Design review of the part built by this model. Coordinates are the model's own, in mm. A direction names the side the tool comes from. Round coordinates to 2 decimals unless told otherwise and drop trailing zeros. Loops run counter-clockwise (first coordinate to the right, second up) from the corner with the lowest first, then second, coordinate; pieces in that order, holes last. Notation, with made-up numbers: (36, 89) - (56, 89) arc R24 ccw to (56, 110) - close; hole circle Ø3 at (75, 78.5). An arc over 180 degrees is marked (long way). Answer as CSV lines item,"result". Start each with the question number.
(1) Consider section A-A (x = 23.75). Give the boundary of the cut face in (y, z), and give its area (3 significant figures).
(2) Consider section B-B (z = -1.75). Give the boundary of the cut face in (x, y), and give its area (3 significant figures).
(3) Consider section C-C (y = -14.25). Give the boundary of the cut face in (x, z).
(4) Mouldability with a two-part tool opening along X and no side actions: class faces 5 (the cylindrical face through (-21.461, -3.074, -0.14)), 6 (the flat face through (26, -3, 0)), 7 (the flat face through (11, -5, -7)) as released by +X, released by -X, zero draft, split by the parting line, or undercut.
(5) For P1, Ø3, axis at x = -9.5, z = -5.5, coming from the +Y side; P2, Ø2, axis at y = -22, z = 0.5, coming from the -X side; P3, Ø1, axis at x = 15.5, z = -3, coming from the +Y side; P4, Ø1.5, axis at x = -13, z = -8, coming from the -Y side, all flat-tipped, find the tip position at first contact; note any pin that passes through.
(6) For faces 1 (the flat face through (0, -25, 0)), 2 (the flat face through (-14, -8, 8)), 3 (the cylindrical face through (-5.85, -5.57, -7.46)), 4 (the flat face through (-7, -12, 0)), list the 3-axis set-ups (+Z, -Z, +X, -X, +Y, -Y) from which the entire face can be reached by the end or side of a thin tool; tool diameter is ignored.
(7) Consider section D-D (x = -23). Give the boundary of the cut face in (y, z).
(8) Wall thickness on L1, parallel to Z at x = -23.75, y = -1.7; L2, parallel to X at y = -1.15, z = -4.75; L3, parallel to X at y = -15.5, z = 4: over which ranges is each line inside the solid? List them lowest first.
from build123d import *

# Parameters (mm, degrees)
BOSS_EXTRUDE1_DEPTH = 10
SKETCH2_R           = 2
CUT_EXTRUDE1_DEPTH  = 6
SKETCH3_W           = 10
SKETCH3_H           = 12
CUT_EXTRUDE2_DEPTH  = 21
FILLET1_R           = 2


with BuildPart() as part:
    # Sketch1 → Boss-Extrude1 (new, symmetric)
    with BuildSketch(Plane.XY):
        Polygon((-30, 0), (-17, 0), (-17, -5), (-5.25, -5), (-5.25, -22), (5.25, -22), (5.25, -5), (17, -5), (17, 0), (30, 0), (30, -3), (20, -3), (20, -8), (8.25, -8), (8.25, -25), (-8.25, -25), (-8.25, -8), (-20, -8), (-20, -3), (-30, -3), align=None)
    extrude(amount=BOSS_EXTRUDE1_DEPTH, both=True)

    # Sketch2 → Cut-Extrude1 (cut)
    with BuildSketch(Plane(origin=(0, 0, 0), x_dir=(1, 0, 0), z_dir=(0, 1, 0))):
        with Locations(Location((-23.75, 4.75, 0), (0, 0, 270))):
            Circle(SKETCH2_R)
        with Locations(Location((-23.75, -4.75, 0), (0, 0, 270))):
            Circle(SKETCH2_R)
        with Locations(Location((23.75, 4.75, 0), (0, 0, 270))):
            Circle(SKETCH2_R)
        with Locations(Location((23.75, -4.75, 0), (0, 0, 270))):
            Circle(SKETCH2_R)
    extrude(amount=-CUT_EXTRUDE1_DEPTH, mode=Mode.SUBTRACT)

    # Sketch3 → Cut-Extrude2 (cut, symmetric)
    with BuildSketch(Plane(origin=(0, 0, 0), x_dir=(0, 0, -1), z_dir=(1, 0, 0))):
        with Locations((0, -6)):
            Rectangle(SKETCH3_W, SKETCH3_H)
    extrude(amount=CUT_EXTRUDE2_DEPTH, both=True, mode=Mode.SUBTRACT)

    # Fillet1
    # the kernel refuses this fillet: 2 mm, written as the material it adds along each edge
    with BuildSketch(Plane(origin=(-17, -5, 10), x_dir=(0, 1, 0), z_dir=(0, 0, -1)), Plane(origin=(17, -5, 10), x_dir=(-1, 0, 0), z_dir=(0, 0, -1)), Plane(origin=(8.25, -8, 10), x_dir=(1, 0, 0), z_dir=(0, 0, -1)), Plane(origin=(-8.25, -8, 10), x_dir=(0, -1, 0), z_dir=(0, 0, -1)), Plane(origin=(-17, -5, -5), x_dir=(0, 1, 0), z_dir=(0, 0, -1)), Plane(origin=(17, -5, -5), x_dir=(-1, 0, 0), z_dir=(0, 0, -1)), Plane(origin=(-8.25, -8, -5), x_dir=(0, -1, 0), z_dir=(0, 0, -1))) as fillet1_piece_1:
        with BuildLine():
            CenterArc((FILLET1_R, FILLET1_R), FILLET1_R, 180, 90)
            Line((0, FILLET1_R), (0, 0))
            Line((0, 0), (FILLET1_R, 0))
        make_face()
    extrude(amount=5)
    with BuildSketch(Plane(origin=(-5.25, -22, 10), x_dir=(0, 1, 0), z_dir=(0, 0, -1)), Plane(origin=(5.25, -22, 10), x_dir=(-1, 0, 0), z_dir=(0, 0, -1))) as fillet1_piece_2:
        with BuildLine():
            CenterArc((FILLET1_R, FILLET1_R), FILLET1_R, 180, 90)
            Line((0, FILLET1_R), (0, 0))
            Line((0, 0), (FILLET1_R, 0))
        make_face()
    extrude(amount=20)
    with BuildSketch(Plane(origin=(20, -3, 10), x_dir=(1, 0, 0), z_dir=(0, 0, -1))) as fillet1_piece_3_section:
        with BuildLine():
            CenterArc((FILLET1_R, FILLET1_R), FILLET1_R, 180, 90)
            Line((0, FILLET1_R), (0, 0))
            Line((0, 0), (FILLET1_R, 0))
        make_face()
    fillet1_piece_3 = extrude(amount=5, mode=Mode.PRIVATE)
    fillet1_piece_3 = split(fillet1_piece_3, bisect_by=Plane(origin=(21, -3.048479196, 7.515597856), z_dir=(1, 0, 0)), keep=Keep.TOP, mode=Mode.PRIVATE)
    fillet1_piece_3 = fillet1_piece_3 - Plane(origin=(23.75, -3.048479196, 4.75), x_dir=(0, 0, 1), z_dir=(0, 1, 0)) * Cylinder(2, 18, mode=Mode.PRIVATE)
    add(fillet1_piece_3)
    with BuildSketch(Plane(origin=(20, -3, 10), x_dir=(1, 0, 0), z_dir=(0, 0, -1))) as fillet1_piece_4_section:
        with BuildLine():
            CenterArc((FILLET1_R, FILLET1_R), FILLET1_R, 180, 90)
            Line((0, FILLET1_R), (0, 0))
            Line((0, 0), (FILLET1_R, 0))
        make_face()
    fillet1_piece_4 = extrude(amount=5, mode=Mode.PRIVATE)
    fillet1_piece_4 = split(fillet1_piece_4, bisect_by=Plane(origin=(21, -3.51024012, 7.5), z_dir=(-1, 0, 0)), keep=Keep.TOP, mode=Mode.PRIVATE)
    add(fillet1_piece_4)
    with BuildSketch(Plane(origin=(20, -3, 10), x_dir=(1, 0, 0), z_dir=(0, 0, -1))) as fillet1_piece_5_section:
        with BuildLine():
            CenterArc((FILLET1_R, FILLET1_R), FILLET1_R, 180, 90)
            Line((0, FILLET1_R), (0, 0))
            Line((0, 0), (FILLET1_R, 0))
        make_face()
    fillet1_piece_5 = extrude(amount=10, mode=Mode.PRIVATE)
    fillet1_piece_5 = split(fillet1_piece_5, bisect_by=Plane(origin=(21.317615257, -3.049059645, 5), z_dir=(0, 0, -1)), keep=Keep.TOP, mode=Mode.PRIVATE)
    fillet1_piece_5 = split(fillet1_piece_5, bisect_by=Plane(origin=(21, -3.049059645, 2.467907611), z_dir=(1, 0, 0)), keep=Keep.TOP, mode=Mode.PRIVATE)
    fillet1_piece_5 = fillet1_piece_5 - Plane(origin=(23.75, -3.049059645, 4.75), x_dir=(0, 0, 1), z_dir=(0, 1, 0)) * Cylinder(2, 28, mode=Mode.PRIVATE)
    add(fillet1_piece_5)
    with BuildSketch(Plane(origin=(-20, -3, 0), x_dir=(-1, 0, 0), z_dir=(0, 0, 1))) as fillet1_piece_6_section:
        with BuildLine():
            CenterArc((FILLET1_R, FILLET1_R), FILLET1_R, 180, 90)
            Line((0, FILLET1_R), (0, 0))
            Line((0, 0), (FILLET1_R, 0))
        make_face()
    fillet1_piece_6 = extrude(amount=10, mode=Mode.PRIVATE)
    fillet1_piece_6 = split(fillet1_piece_6, bisect_by=Plane(origin=(-21.317615257, -3.049059645, 5), z_dir=(0, 0, -1)), keep=Keep.TOP, mode=Mode.PRIVATE)
    fillet1_piece_6 = split(fillet1_piece_6, bisect_by=Plane(origin=(-21, -3.049059645, 2.46790761), z_dir=(-1, 0, 0)), keep=Keep.TOP, mode=Mode.PRIVATE)
    fillet1_piece_6 = fillet1_piece_6 - Plane(origin=(-23.75, -3.049059645, 4.75), x_dir=(0, 0, 1), z_dir=(0, 1, 0)) * Cylinder(2, 28, mode=Mode.PRIVATE)
    add(fillet1_piece_6)
    with BuildSketch(Plane(origin=(-20, -3, 5), x_dir=(-1, 0, 0), z_dir=(0, 0, 1))) as fillet1_piece_7_section:
        with BuildLine():
            CenterArc((FILLET1_R, FILLET1_R), FILLET1_R, 180, 90)
            Line((0, FILLET1_R), (0, 0))
            Line((0, 0), (FILLET1_R, 0))
        make_face()
    fillet1_piece_7 = extrude(amount=5, mode=Mode.PRIVATE)
    fillet1_piece_7 = split(fillet1_piece_7, bisect_by=Plane(origin=(-21, -3.048479196, 7.515597855), z_dir=(-1, 0, 0)), keep=Keep.TOP, mode=Mode.PRIVATE)
    fillet1_piece_7 = fillet1_piece_7 - Plane(origin=(-23.75, -3.048479196, 4.75), x_dir=(0, 0, 1), z_dir=(0, 1, 0)) * Cylinder(2, 18, mode=Mode.PRIVATE)
    add(fillet1_piece_7)
    with BuildSketch(Plane(origin=(-20, -3, 5), x_dir=(-1, 0, 0), z_dir=(0, 0, 1))) as fillet1_piece_8_section:
        with BuildLine():
            CenterArc((FILLET1_R, FILLET1_R), FILLET1_R, 180, 90)
            Line((0, FILLET1_R), (0, 0))
            Line((0, 0), (FILLET1_R, 0))
        make_face()
    fillet1_piece_8 = extrude(amount=5, mode=Mode.PRIVATE)
    fillet1_piece_8 = split(fillet1_piece_8, bisect_by=Plane(origin=(-21, -3.51024012, 7.5), z_dir=(1, 0, 0)), keep=Keep.TOP, mode=Mode.PRIVATE)
    add(fillet1_piece_8)
    with BuildSketch(Plane(origin=(20, -3, 0), x_dir=(1, 0, 0), z_dir=(0, 0, -1))) as fillet1_piece_9_section:
        with BuildLine():
            CenterArc((FILLET1_R, FILLET1_R), FILLET1_R, 180, 90)
            Line((0, FILLET1_R), (0, 0))
            Line((0, 0), (FILLET1_R, 0))
        make_face()
    fillet1_piece_9 = extrude(amount=10, mode=Mode.PRIVATE)
    fillet1_piece_9 = split(fillet1_piece_9, bisect_by=Plane(origin=(21, -3.049059645, -2.46790761), z_dir=(1, 0, 0)), keep=Keep.TOP, mode=Mode.PRIVATE)
    fillet1_piece_9 = split(fillet1_piece_9, bisect_by=Plane(origin=(21.317615257, -3.049059645, -5), z_dir=(0, 0, 1)), keep=Keep.TOP, mode=Mode.PRIVATE)
    fillet1_piece_9 = fillet1_piece_9 - Plane(origin=(23.75, -3.049059645, -4.75), x_dir=(0, 0, 1), z_dir=(0, 1, 0)) * Cylinder(2, 28, mode=Mode.PRIVATE)
    add(fillet1_piece_9)
    with BuildSketch(Plane(origin=(20, -3, -5), x_dir=(1, 0, 0), z_dir=(0, 0, -1))) as fillet1_piece_10_section:
        with BuildLine():
            CenterArc((FILLET1_R, FILLET1_R), FILLET1_R, 180, 90)
            Line((0, FILLET1_R), (0, 0))
            Line((0, 0), (FILLET1_R, 0))
        make_face()
    fillet1_piece_10 = extrude(amount=5, mode=Mode.PRIVATE)
    fillet1_piece_10 = split(fillet1_piece_10, bisect_by=Plane(origin=(21, -3.048479196, -7.515597854), z_dir=(1, 0, 0)), keep=Keep.TOP, mode=Mode.PRIVATE)
    fillet1_piece_10 = fillet1_piece_10 - Plane(origin=(23.75, -3.048479196, -4.75), x_dir=(0, 0, 1), z_dir=(0, 1, 0)) * Cylinder(2, 18, mode=Mode.PRIVATE)
    add(fillet1_piece_10)
    with BuildSketch(Plane(origin=(20, -3, -5), x_dir=(1, 0, 0), z_dir=(0, 0, -1))) as fillet1_piece_11_section:
        with BuildLine():
            CenterArc((FILLET1_R, FILLET1_R), FILLET1_R, 180, 90)
            Line((0, FILLET1_R), (0, 0))
            Line((0, 0), (FILLET1_R, 0))
        make_face()
    fillet1_piece_11 = extrude(amount=5, mode=Mode.PRIVATE)
    fillet1_piece_11 = split(fillet1_piece_11, bisect_by=Plane(origin=(21, -3.51024012, -7.5), z_dir=(-1, 0, 0)), keep=Keep.TOP, mode=Mode.PRIVATE)
    add(fillet1_piece_11)
    with BuildSketch(Plane(origin=(8.25, -8, -5), x_dir=(0, -1, 0), z_dir=(0, 0, -1))) as fillet1_piece_12:
        with BuildLine():
            CenterArc((FILLET1_R, -FILLET1_R), FILLET1_R, 90, 90)
            Line((0, -FILLET1_R), (0, 0))
            Line((0, 0), (FILLET1_R, 0))
        make_face()
    extrude(amount=5)
    with BuildSketch(Plane(origin=(-20, -3, -10), x_dir=(-1, 0, 0), z_dir=(0, 0, 1))) as fillet1_piece_13_section:
        with BuildLine():
            CenterArc((FILLET1_R, FILLET1_R), FILLET1_R, 180, 90)
            Line((0, FILLET1_R), (0, 0))
            Line((0, 0), (FILLET1_R, 0))
        make_face()
    fillet1_piece_13 = extrude(amount=5, mode=Mode.PRIVATE)
    fillet1_piece_13 = split(fillet1_piece_13, bisect_by=Plane(origin=(-21, -3.048479196, -7.515597855), z_dir=(-1, 0, 0)), keep=Keep.TOP, mode=Mode.PRIVATE)
    fillet1_piece_13 = fillet1_piece_13 - Plane(origin=(-23.75, -3.048479196, -4.75), x_dir=(0, 0, 1), z_dir=(0, 1, 0)) * Cylinder(2, 18, mode=Mode.PRIVATE)
    add(fillet1_piece_13)
    with BuildSketch(Plane(origin=(-20, -3, -10), x_dir=(-1, 0, 0), z_dir=(0, 0, 1))) as fillet1_piece_14_section:
        with BuildLine():
            CenterArc((FILLET1_R, FILLET1_R), FILLET1_R, 180, 90)
            Line((0, FILLET1_R), (0, 0))
            Line((0, 0), (FILLET1_R, 0))
        make_face()
    fillet1_piece_14 = extrude(amount=5, mode=Mode.PRIVATE)
    fillet1_piece_14 = split(fillet1_piece_14, bisect_by=Plane(origin=(-21, -3.51024012, -7.5), z_dir=(1, 0, 0)), keep=Keep.TOP, mode=Mode.PRIVATE)
    add(fillet1_piece_14)
    with BuildSketch(Plane(origin=(-20, -3, -10), x_dir=(-1, 0, 0), z_dir=(0, 0, 1))) as fillet1_piece_15_section:
        with BuildLine():
            CenterArc((FILLET1_R, FILLET1_R), FILLET1_R, 180, 90)
            Line((0, FILLET1_R), (0, 0))
            Line((0, 0), (FILLET1_R, 0))
        make_face()
    fillet1_piece_15 = extrude(amount=10, mode=Mode.PRIVATE)
    fillet1_piece_15 = split(fillet1_piece_15, bisect_by=Plane(origin=(-21, -3.049059645, -2.467907611), z_dir=(-1, 0, 0)), keep=Keep.TOP, mode=Mode.PRIVATE)
    fillet1_piece_15 = split(fillet1_piece_15, bisect_by=Plane(origin=(-21.317615257, -3.049059645, -5), z_dir=(0, 0, 1)), keep=Keep.TOP, mode=Mode.PRIVATE)
    fillet1_piece_15 = fillet1_piece_15 - Plane(origin=(-23.75, -3.049059645, -4.75), x_dir=(0, 0, 1), z_dir=(0, 1, 0)) * Cylinder(2, 28, mode=Mode.PRIVATE)
    add(fillet1_piece_15)
    # the kernel refuses this fillet: 2 mm, written as the material it takes off along each edge
    with BuildSketch(Plane(origin=(-17, 0, 15), x_dir=(-1, 0, 0), z_dir=(0, 0, -1)), Plane(origin=(20, -8, 15), x_dir=(0, 1, 0), z_dir=(0, 0, -1)), Plane(origin=(-20, -8, 15), x_dir=(1, 0, 0), z_dir=(0, 0, -1)), Plane(origin=(-17, 0, 0), x_dir=(-1, 0, 0), z_dir=(0, 0, -1)), Plane(origin=(5.25, -5, 0), x_dir=(0, -1, 0), z_dir=(0, 0, -1))) as fillet1_2_piece_1:
        with BuildLine():
            CenterArc((FILLET1_R, -FILLET1_R), FILLET1_R, 90, 90)
            Line((0, -FILLET1_R), (0, 0))
            Line((0, 0), (FILLET1_R, 0))
        make_face()
    extrude(amount=15, mode=Mode.SUBTRACT)
    with BuildSketch(Plane(origin=(-5.25, -5, 15), x_dir=(0, -1, 0), z_dir=(0, 0, -1)), Plane(origin=(5.25, -5, 15), x_dir=(1, 0, 0), z_dir=(0, 0, -1)), Plane(origin=(17, 0, 15), x_dir=(1, 0, 0), z_dir=(0, 0, -1)), Plane(origin=(-5.25, -5, 0), x_dir=(0, -1, 0), z_dir=(0, 0, -1)), Plane(origin=(17, 0, 0), x_dir=(1, 0, 0), z_dir=(0, 0, -1)), Plane(origin=(20, -8, 0), x_dir=(-1, 0, 0), z_dir=(0, 0, -1)), Plane(origin=(-20, -8, 0), x_dir=(0, 1, 0), z_dir=(0, 0, -1))) as fillet1_2_piece_2:
        with BuildLine():
            CenterArc((FILLET1_R, FILLET1_R), FILLET1_R, 180, 90)
            Line((0, FILLET1_R), (0, 0))
            Line((0, 0), (FILLET1_R, 0))
        make_face()
    extrude(amount=15, mode=Mode.SUBTRACT)
    with BuildSketch(Plane(origin=(8.25, -25, 15), x_dir=(-1, 0, 0), z_dir=(0, 0, -1)), Plane(origin=(-8.25, -25, 15), x_dir=(0, 1, 0), z_dir=(0, 0, -1)), Plane(origin=(-30, -3, -15), x_dir=(1, 0, 0), z_dir=(0, 0, 1))) as fillet1_2_piece_3:
        with BuildLine():
            CenterArc((FILLET1_R, FILLET1_R), FILLET1_R, 180, 90)
            Line((0, FILLET1_R), (0, 0))
            Line((0, 0), (FILLET1_R, 0))
        make_face()
    extrude(amount=30, mode=Mode.SUBTRACT)


solid = part.part
Determined:
1,outline,"(-3, -10) - (0, -10) - (0, -6.75) - (-3, -6.75) - close; (-3, -2.75) - (0, -2.75) - (0, 2.75) - (-3, 2.75) - close; (-3, 6.75) - (0, 6.75) - (0, 10) - (-3, 10) - close"
1,area,"36.0 mm^2"
2,outline,"(-30, -1) arc R2 ccw to (-28, -3) - (-22, -3) arc R2 cw to (-21, -3.27) - (-21, 0) - (-30, 0) - close; (-8.25, -23) arc R2 ccw to (-6.25, -25) - (6.25, -25) arc R2 ccw to (8.25, -23) - (8.25, -12) - (5.25, -12) - (5.25, -20) arc R2 cw to (3.25, -22) - (-3.25, -22) arc R2 cw to (-5.25, -20) - (-5.25, -12) - (-8.25, -12) - close; (21, -3.27) arc R2 cw to (22, -3) - (30, -3) - (30, 0) - (21, 0) - close"
2,area,"163 mm^2"
3,outline,"(-8.25, -10) - (-5.25, -10) - (-5.25, 10) - (-8.25, 10) - close; (5.25, -10) - (8.25, -10) - (8.25, 10) - (5.25, 10) - close"
4,face 5,"released by -X"
4,face 6,"zero draft"
4,face 7,"undercut"
5,P1,"stops at y = -5"
5,P2,"stops at x = -8.25"
5,P3,"passes through"
5,P4,"stops at y = -8"
6,face 1,"+Z, -Z, +X, -X, -Y"
6,face 2,"+Z, -Z, -X, -Y"
6,face 3,"+Z, -Z, +Y"
6,face 4,"+X, -X, +Y"
7,outline,"(-3, -10) - (0, -10) - (0, -6.6) - (-3, -6.6) - close; (-3, -2.9) - (0, -2.9) - (0, 2.9) - (-3, 2.9) - close; (-3, 6.6) - (0, 6.6) - (0, 10) - (-3, 10) - close"
8,L1,"z = -10 to -6.75, -2.75 to 2.75, 6.75 to 10"
8,L2,"x = -29.99 to -25.75, -21.75 to -21, 21 to 21.75, 25.75 to 30"
8,L3,"x = -8.25 to -5.25, 5.25 to 8.25"
